Autodesk Inventor part; units mm, degrees
ref_plane "YZ Plane" through (0, 0, 0) normal (1, 0, 0) x (0, 1, 0)
ref_plane "XZ Plane" through (0, 0, 0) normal (0, 1, 0) x (-1, 0, 0)
ref_plane "XY Plane" through (0, 0, 0) normal (0, 0, 1) x (1, 0, 0)
sketch "Sketch1" plane through (0, 0, 0) normal (0, 1, 0) x (-1, 0, 0)
  line L0 (0, 0) -> (11.557, 0)
  line L1 (11.557, 0) -> (11.557, -19.177)
  line L2 (11.557, -19.177) -> (0, -19.177)
  line L3 (0, -19.177) -> (0, 0)
  line L4 (3.175, -3.175) -> (8.382, -3.175)
  line L5 (8.382, -3.175) -> (8.382, -16.002)
  line L6 (8.382, -16.002) -> (3.175, -16.002)
  line L7 (3.175, -16.002) -> (3.175, -3.175)
  line L8 (8.382, -3.175) -> (5.969, -3.175)
  line L9 (5.969, -3.175) -> (5.969, -5.588)
  line L10 (5.969, -5.588) -> (8.382, -5.588)
  line L11 (8.382, -5.588) -> (8.382, -3.175)
  dimension "d0" = 12.827
  dimension "d1" = 5.207
  dimension "d2" = 3.175
  dimension "d3" = 3.175
  dimension "d4" = 3.175
  dimension "d5" = 3.175
  dimension "d6" = 2.413
  dimension "d7" = 2.413
extrude "Extrusion1" add sketch "Sketch1" along normal blind 2.54 contours L0 L1 L2 L3 | L4 L5 L10 L9
sketch "Sketch2" plane through (0, 2.54, 0) normal (0, 1, 0) x (1, 0, 0)
  line L0 (-8.382, 5.588) -> (-8.382, 16.002) construction
  line L1 (-8.382, 16.002) -> (-3.175, 16.002) construction
  line L2 (-3.175, 16.002) -> (-3.175, 3.175) construction
  line L3 (-3.175, 3.175) -> (-5.969, 3.175) construction
  line L4 (-5.969, 3.175) -> (-5.969, 5.588) construction
  line L5 (-5.969, 5.588) -> (-8.382, 5.588) construction
  line L6 (-11.557, 19.177) -> (-11.557, 0)
  line L7 (-11.557, 0) -> (0, 0)
  line L8 (0, 0) -> (0, 19.177)
  line L9 (0, 19.177) -> (-11.557, 19.177)
  line L10 (-9.906, 1.651) -> (-1.651, 1.651)
  line L11 (-1.651, 1.651) -> (-1.651, 17.526)
  line L12 (-1.651, 17.526) -> (-9.906, 17.526)
  line L13 (-9.906, 17.526) -> (-9.906, 1.651)
  dimension "d10" = 1.524
  dimension "d11" = 1.524
  dimension "d14" = 1.524
  dimension "d15" = 1.524
extrude "Extrusion2" add sketch "Sketch2" along normal blind 6.35
fillet "Fillet1" radius 0.635 8 edges at (0, 4.445, 0) (-11.557, 4.445, 0) (-11.557, 4.445, -19.177) (0, 4.445, -19.177) (-9.906, 5.715, -17.526) (-9.906, 5.715, -1.651) (-1.651, 5.715, -17.526) (-1.651, 5.715, -1.651)
equation "\"d3\" = d2"
equation "\"d4\" = d2"
equation "\"d5\" = d4"
equation "\"d11\" = d10"
equation "\"d14\" = d10"
equation "\"d15\" = d10"
properties part number "ForeConnectorHousing" material "ABS Plastic"
CAD build for the part. Positions are in the model's coordinates, mm. A direction names the side the tool comes from. Round coordinates to 2 decimals unless told otherwise and drop trailing zeros. Write each loop counter-clockwise with the first axis right and the second up, starting at its lowest first coordinate (ties: lowest second). Pieces come first, ordered by that corner, then holes. Notation, with made-up numbers: M 1,-15 L 54,-15 A19 cw 54,20 Z; hole C 8.25,-25.75 d3. An arc over 180 degrees is marked long. Use a Markdown table: item, result. Add a question column.
1. Slice it at B-B on z = -6.25. Give the cut face in (x, y) (3 decimals).
2. Drill centre lines: probe 1 along Z at (x, y) = (-3, 4.75); probe 2 along Z at (x, y) = (-4.75, 1.5) (3 decimals); probe 3 along X at (y, z) = (7.25, -16.5). Where is each one in solid material? Low to high.
3. Slice it at D-D on x = -9. Give the cut face in (y, z).
4. 3-axis set-ups, long thin cutter, end or side, ignore diameter. For faces 5 (the face through (-3.175, 1, -10)), 6 (the face through (-9.906, 6, -10)), 7 (the face through (-11.557, 4, -10)): which of +Z, -Z, +X, -X, +Y, -Y reach the whole face in a straight line?
5. Pull direction X, two halves, no side cores. Call faces 1 (the face through (-6, 6, -1.651)), 2 (the face through (-7, 1, -5.588)), 3 (the face through (0, 4, -9)), 4 (the face through (-6, 4, 0)): released by +X, released by -X, zero draft, split by the parting line, or undercut.
6. Slice it at A-A on y = 1.75. Give the cut face in (x, z) (3 decimals).
7. Slice it at C-C on x = -4. Give the cut face in (y, z) (3 decimals).
Reply:
| question | item | result |
|---|---|---|
| 1 | outline | M -11.557,0 L -8.382,0 L -8.382,2.54 L -9.906,2.54 L -9.906,8.89 L -11.557,8.89 Z; M -3.175,0 L 0,0 L 0,8.89 L -1.651,8.89 L -1.651,2.54 L -3.175,2.54 Z |
| 2 | probe 1 | z = -19.18 to -17.53, -1.65 to 0 |
| 2 | probe 2 | z = -19.177 to -16.002, -3.175 to 0 |
| 2 | probe 3 | x = -11.56 to -9.91, -1.65 to 0 |
| 3 | outline | M 0,-19.18 L 8.89,-19.18 L 8.89,-17.53 L 2.54,-17.53 L 2.54,-1.65 L 8.89,-1.65 L 8.89,0 L 0,0 Z |
| 4 | face 5 | +Y, -Y |
| 4 | face 6 | +Y |
| 4 | face 7 | +Z, -Z, -X, +Y, -Y |
| 5 | face 1 | undercut |
| 5 | face 2 | undercut |
| 5 | face 3 | released by +X |
| 5 | face 4 | zero draft |
| 6 | outline | M -11.557,-18.542 A0.635 ccw -10.922,-19.177 L -0.635,-19.177 A0.635 ccw 0,-18.542 L 0,-0.635 A0.635 ccw -0.635,0 L -10.922,0 A0.635 ccw -11.557,-0.635 Z; hole M -8.382,-16.002 L -3.175,-16.002 L -3.175,-3.175 L -5.969,-3.175 L -5.969,-5.588 L -8.382,-5.588 Z |
| 7 | outline | M 0,-19.177 L 8.89,-19.177 L 8.89,-17.526 L 2.54,-17.526 L 2.54,-16.002 L 0,-16.002 Z; M 0,-3.175 L 2.54,-3.175 L 2.54,-1.651 L 8.89,-1.651 L 8.89,0 L 0,0 Z |
